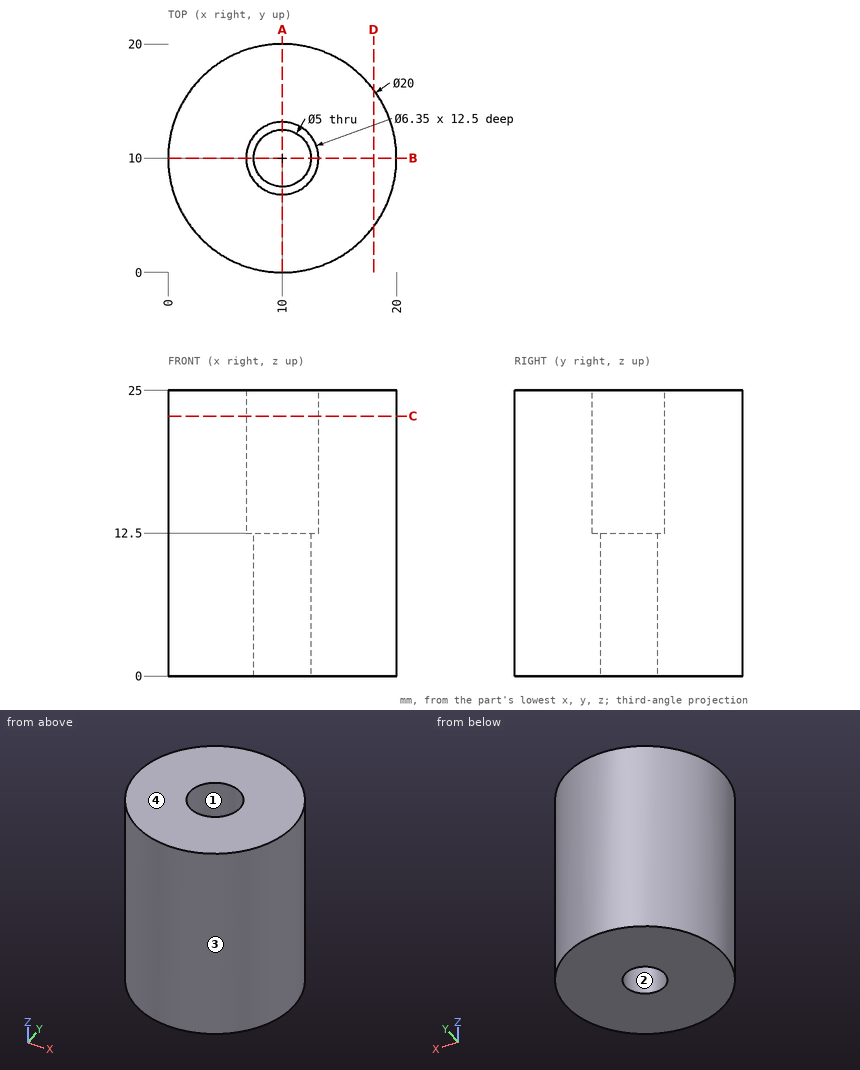
For this review, use the dimensioned drawing (mm, ordinates from the lowest corner) and the shaded views. Round coordinates to 2 decimals unless told otherwise and drop trailing zeros. Loops run counter-clockwise (first coordinate to the right, second up) from the corner with the lowest first, then second, coordinate; pieces in that order, holes last. Notation, with made-up numbers: (-17, 50) -> (34, 50) arc R28 cw to (34, 80) -> close; hole circle Ø2 at (77.25, -12). An arc over 180 degrees is marked (long way). Write item = value, one per line. Start each with the question number.
Item 1: Take a section at A-A on x = 10. Give the boundary of the cut face in (y, z) (3 decimals).
Item 2: Mouldability with a two-part tool opening along Y and no side actions: class the marked faces 1, 2, 3 and 4 as released by +Y, released by -Y, zero draft, split by the parting line, or undercut.
Item 3: Take a section at D-D on x = 18. Give the boundary of the cut face in (y, z), plus the area to 3 significant figures.
Item 4: Take a section at C-C on z = 22.75. Give the boundary of the cut face in (x, y) (3 decimals).
Item 5: To check wall thickness, follow L1, parallel to Y at x = 10, z = 9.25; L2, parallel to Y at x = 10, z = 22 (3 decimals); L3, parallel to Y at x = 6.5, z = 14.25. State the ranges of each line that lie inside material, in increasing order.
Item 6: Insertion check: pin 1 (6 mm diameter, centred on x = 14, z = 9, fed in from +Y); pin 2 (2 mm diameter, centred on x = 14.5, z = 3, fed in from -Y); pin 3 (4 mm diameter, centred on x = 10, y = 10, fed in from -Z); pin 4 (1.5 mm diameter, centred on x = 9, z = 20.5, fed in from -Y). Each pin has a flat end and moves straight along its axis. Give the tip position at first contact, or say it passes through.
Result:
q1.outline = (0, 0) -> (7.5, 0) -> (7.5, 12.5) -> (6.825, 12.5) -> (6.825, 25) -> (0, 25) -> close; (12.5, 0) -> (20, 0) -> (20, 25) -> (13.175, 25) -> (13.175, 12.5) -> (12.5, 12.5) -> close
q2.face_1 = undercut
q2.face_2 = undercut
q2.face_3 = split by the parting line
q2.face_4 = zero draft
q3.outline = (4, 0) -> (16, 0) -> (16, 25) -> (4, 25) -> close
q3.area = 300 mm²
q4.outline = circle Ø20 at (10, 10); hole circle Ø6.35 at (10, 10)
q5.L1 = 0 to 7.5, 12.5 to 20
q5.L2 = 0 to 6.825, 13.175 to 20
q5.L3 = 0.63 to 19.37
q6.pin_1 = 19.95
q6.pin_2 = 0.63
q6.pin_3 = through
q6.pin_4 = 0
